Check sheet for the modelled part. Datum: model origin and axes. Units: mm. A direction names the side the tool comes from. Give positions to 0.01 mm unless a question says otherwise; leave off trailing zeros. Order: outer loops, then holes, each group sorted by start corner. A loop starts at its lowest first (then second) coordinate and runs counter-clockwise, first axis right, second up.
Item 1: Release check for a two-part mould opening along Y. For faces 3 (the cylindrical face through (-8.73, 5.03, 3.54)), 4 (the flat face through (8.994, 0, 4)), 5 (the cylindrical face through (0.015, -10.076, 3.662)), 6 (the flat face through (-7.794, 0, 4)) record: released by +Y, released by -Y, zero draft, split by the parting line, or undercut.
Item 2: Sectioned sample at B-B on y = 2.5. Record the boundary of the cut face in (x, z).
Item 3: Gauge pin test, flat ends, axial feed: P1, Ø1.5, axis at x = 1.5, y = 1.5, coming from the +Z side; P2, Ø4, axis at x = 2.5, z = 1, coming from the +Y side. Record the tip position at first contact, or that the pin passes through.
Item 4: Material ranges on line 1 along X through (y, z) = (4, 0.5); line 2 along Z through (x, y) = (-7.5, -0.5); line 3 along X through (y, z) = (7.5, 1.75), recorded low to high.
Item 5: Access from +Z, -Z, +X, -X, +Y, -Y to the whole of each face (thin tool, end or side, straight path). Record for faces 1 (the flat face through (0, 0, -0.8)), 2 (the flat face through (7.794, 0, 4)).
Item 6: Sectioned sample at C-C on x = 3.75. Record the boundary of the cut face in (y, z).
Item 7: Sectioned sample at A-A on z = 7. Record the boundary of the cut face in (x, y), and give its area (3 significant figures).
from build123d import *

# Parameters (mm, degrees)
F1_DEPTH = 8
F2_DEPTH = 0.8
F3_R     = 2


with BuildPart() as f1:
    # F0 (on Top) → F1 (new body)
    with BuildSketch(Plane.XY):
        Polygon((-8.9942286341, 5.192820323), (-8.9942286341, -5.192820323), (0, -10.3856406461), (8.9942286341, -5.192820323), (8.9942286341, 5.192820323), (0, 10.3856406461), align=None)
        Polygon((0, -9), (-7.7942286341, -4.5), (-7.7942286341, 4.5), (0, 9), (7.7942286341, 4.5), (7.7942286341, -4.5), align=None, mode=Mode.SUBTRACT)
    extrude(amount=F1_DEPTH)

    # F0 (on Top) → F2 (join)
    with BuildSketch(Plane.XY):
        Polygon((-8.9942286341, 5.192820323), (-8.9942286341, -5.192820323), (0, -10.3856406461), (8.9942286341, -5.192820323), (8.9942286341, 5.192820323), (0, 10.3856406461), align=None)
        Polygon((0, -9), (-7.7942286341, -4.5), (-7.7942286341, 4.5), (0, 9), (7.7942286341, 4.5), (7.7942286341, -4.5), align=None, mode=Mode.SUBTRACT)
        Polygon((-7.7942286341, 4.5), (-7.7942286341, -4.5), (0, -9), (7.7942286341, -4.5), (7.7942286341, 4.5), (0, 9), align=None)
    extrude(amount=-F2_DEPTH)

    # F3
    f3_edges = [f1.edges().sort_by_distance(p)[0] for p in [
        (-8.994229, -5.19282, 3.6),
        (-8.994229, 5.19282, 3.6),
        (0, -10.385641, 3.6),
        (8.994229, -5.19282, 3.6),
        (8.994229, 5.19282, 3.6),
        (0, 10.385641, 3.6),
    ]]
    fillet(f3_edges, radius=F3_R)


solid = f1.part
Report:
1. face 3: released by +Y
1. face 4: zero draft
1. face 5: released by -Y
1. face 6: undercut
2. outline: (-8.99, -0.8) - (8.99, -0.8) - (8.99, 8) - (7.79, 8) - (7.79, 0) - (-7.79, 0) - (-7.79, 8) - (-8.99, 8) - close
3. P1: stops at z = 0
3. P2: stops at y = 10.01
4. line 1: x = -8.99 to -7.79, 7.79 to 8.99
4. line 2: z = -0.8 to 0
4. line 3: x = -5 to -2.6, 2.6 to 5
5. face 1: -Z, +X, -X, +Y, -Y
5. face 2: +Z
6. outline: (-8.22, -0.8) - (8.22, -0.8) - (8.22, 8) - (6.83, 8) - (6.83, 0) - (-6.83, 0) - (-6.83, 8) - (-8.22, 8) - close
7. outline: (-8.99, -4.04) arc R2 ccw to (-7.99, -5.77) - (-1, -9.81) arc R2 ccw to (1, -9.81) - (7.99, -5.77) arc R2 ccw to (8.99, -4.04) - (8.99, 4.04) arc R2 ccw to (7.99, 5.77) - (1, 9.81) arc R2 ccw to (-1, 9.81) - (-7.99, 5.77) arc R2 ccw to (-8.99, 4.04) - close; hole (-7.79, -4.5) - (0, -9) - (7.79, -4.5) - (7.79, 4.5) - (0, 9) - (-7.79, 4.5) - close
7. area: 68.5 mm2
